```python
from build123d import *

# Parameters (mm, degrees)
F0_R          = 0.3175
F1_DEPTH      = 38.1
F1_DEPTH_BACK = 38.1
F0_R_2        = 2.54
F2_DEPTH      = 6.35
F2_DEPTH_BACK = 6.35
F0_R_3        = 4.191
F3_DEPTH      = 5.08
F3_DEPTH_BACK = 5.08


with BuildPart() as f1:
    # F0 (on Top) → F1 (new body, two sides)
    with BuildSketch(Plane.XY) as f1_sk:
        Circle(F0_R)
    extrude(amount=F1_DEPTH)
    extrude(f1_sk.sketch, amount=-F1_DEPTH_BACK)

    # F0 (on Top) → F2 (join, two sides)
    with BuildSketch(Plane.XY) as f2_sk:
        Circle(F0_R_2)
        Circle(F0_R, mode=Mode.SUBTRACT)
    extrude(amount=F2_DEPTH)
    extrude(f2_sk.sketch, amount=-F2_DEPTH_BACK)

    # F0 (on Top) → F3 (join, two sides)
    with BuildSketch(Plane.XY) as f3_sk:
        Circle(F0_R_3)
        Circle(F0_R_2, mode=Mode.SUBTRACT)
    extrude(amount=F3_DEPTH)
    extrude(f3_sk.sketch, amount=-F3_DEPTH_BACK)


solid = f1.part
```
Can you work these out from the model? Positions are in its coordinate system, mm. A direction names the side the tool comes from. Round coordinates to 2 decimals unless told otherwise and drop trailing zeros. Loops run counter-clockwise (first coordinate to the right, second up) from the corner with the lowest first, then second, coordinate; pieces in that order, holes last. Notation, with made-up numbers: M 83,-12 L 133,-12 A36 ccw 133,25 Z; hole C 79.25,-20 d10. An arc over 180 degrees is marked long. Answer in a Markdown table with one row per item.
1. On a 3-axis mill with a long thin cutter (end or side, diameter ignored), from which of +Z, -Z, +X, -X, +Y, -Y can I reach the whole of each face in a straight line? I mean faces 1 (the face through (2, -2, 5.08)), 2 (the face through (3.997, 1.259, 0.071)), 3 (the face through (-0.33, 2.52, -5.71)). Say none if no direction works.
Established:
| item | result |
|---|---|
| face 1 | +Z |
| face 2 | +Z, -Z |
| face 3 | -Z |
2. If we section it at C-C, the plane x = 3.5: Please give me the cut outline in (y, z), plus the area to 3 significant figures.
Established:
| item | result |
|---|---|
| outline | M -2.31,-5.08 L 2.31,-5.08 L 2.31,5.08 L -2.31,5.08 Z |
| area | 46.8 mm² |
3. If we section it at B-B, the plane z = -4: Please give me the cut outline in (x, y), plus the area to 3 significant figures.
Established:
| item | result |
|---|---|
| outline | C 0,0 d8.38 |
| area | 55.2 mm² |
4. If we section it at A-A, the plane y = 1.75: Please give me the cut outline in (x, z), plus the area to 3 significant figures.
Established:
| item | result |
|---|---|
| outline | M -3.81,-5.08 L -1.84,-5.08 L -1.84,-6.35 L 1.84,-6.35 L 1.84,-5.08 L 3.81,-5.08 L 3.81,5.08 L 1.84,5.08 L 1.84,6.35 L -1.84,6.35 L -1.84,5.08 L -3.81,5.08 Z |
| area | 86.7 mm² |
5. I'm going to push flat-ended pins straight in: pin 1 Ø1.5 at (x, y) = (0.5, -0.5) entering from -Z; pin 2 Ø3 at (x, y) = (-3, -0.5) entering from +Z; pin 3 Ø2 at (y, z) = (-1, 23.5) entering from +X; pin 4 Ø3 at (x, y) = (2, 0) entering from -Z. Where does each tip first touch, or does it pass through?
Established:
| item | result |
|---|---|
| pin 1 | z = -38.1 |
| pin 2 | z = 6.35 |
| pin 3 | x = 0.32 |
| pin 4 | z = -6.35 |
6. If we section it at D-D, the plane z = 10: Please give me the cut outline in (x, y) (1 decimal), plus the area to 3 significant figures.
Established:
| item | result |
|---|---|
| outline | C 0,0 d0.6 |
| area | 0.317 mm² |
7. Please list where these lines run through material, in increasing order: line 1 (Y direction, x = 0, z = 18); line 2 (Z direction, x = 3, y = 0.5); line 3 (Z direction, x = -1.5, y = 1). Write a range as from..to.
Established:
| item | result |
|---|---|
| line 1 | -0.32..0.32 |
| line 2 | -5.08..5.08 |
| line 3 | -6.35..6.35 |
